Input: part model. Units: mm. Frame: model coordinates. Coordinates: 2 decimals unless noted, no trailing zeros. Loops run counter-clockwise (first coordinate to the right, second up) from the corner with the lowest first, then second, coordinate; pieces in that order, holes last.
```python
from build123d import *

# Parameters (mm, degrees)
F1_DEPTH = 12.7


# Not quite as in the source:
# - ends of sketch curves that miss each other by under 0.0002 mm in the source are joined


with BuildPart() as f1:
    # F0 (on Front) → F1 (new body)
    with BuildSketch(Plane.XZ):
        with BuildLine():
            Line((-19.0339237452, 12.7), (-38.1, 12.7))
            Line((-38.1, 12.7), (-66.1931892949, 12.6997966278))
            ThreePointArc((-66.1931892949, 12.6997966278), (-78.963911742, 0.170887308), (-66.5349535226, -12.6971318925))
            Line((-66.5349535226, -12.6971318925), (-65.9977308849, -12.6971860797))
            Line((-65.9977308849, -12.6971860797), (-38.1, -12.7))
            Line((-38.1, -12.7), (38.1, -12.7))
            Line((38.1, -12.7), (53.6455512047, -12.7))
            ThreePointArc((53.6455512047, -12.7), (66.3455512047, 0), (53.6455512047, 12.7))
            Line((53.6455512047, 12.7), (38.1, 12.7))
            Line((38.1, 12.7), (-19.0339237452, 12.7))
        make_face()
    extrude(amount=F1_DEPTH)


solid = f1.part
```
Item 1: Line query: L1, parallel to Z at x = -48.5, y = -7.5; L2, parallel to X at y = -7, z = 3; L3, parallel to X at y = -6.75, z = 7.5. Output: solid intervals per line, ascending.
Result:
L1: z = -12.7 to 12.7
L2: x = -78.61 to 65.99
L3: x = -76.51 to 63.89
Item 2: Section query A-A (y = -4.5). Output: boundary loops of the cut face in (x, z).
Result:
outline: (-66.53, -12.7) - (-38.1, -12.7) - (53.65, -12.7) arc R12.7 ccw to (53.65, 12.7) - (-38.1, 12.7) - (-66.19, 12.7) arc R12.7 ccw to start
Item 3: Section query B-B (z = -10.5). Output: boundary loops of the cut face in (x, y), then the cut area to 3 significant figures.
Result:
outline: (-73.41, -12.7) - (60.79, -12.7) - (60.79, 0) - (-73.41, 0) - close
area: 1,700 mm2
Item 4: Contact query for flat-ended pins moving along their axis: P1, Ø12, axis at x = -62.5, z = 9.5, coming from the +Y side; P2, Ø6, axis at y = -5, z = 8.5, coming from the +X side; P3, Ø1.5, axis at y = -3.5, z = 2, coming from the +X side; P4, Ø3, axis at y = -5.5, z = -6, coming from the -X side. Output: stop coordinate, or through.
Result:
P1: stops at y = 0
P2: stops at x = 65.09
P3: stops at x = 66.28
P4: stops at x = -78.14
